Here's how the part is built. I have some questions about the finished solid (model axes, mm). Face numbers are marked on the shaded views. A direction names the side the tool comes from. Round coordinates to 2 decimals unless told otherwise and drop trailing zeros. Write each loop counter-clockwise with the first axis right and the second up, starting at its lowest first coordinate (ties: lowest second). Pieces come first, ordered by that corner, then holes. Notation, with made-up numbers: (77.25, 10) - (87.25, 10) arc R13 cw to (87.25, 20) - close; hole circle Ø2 at (-37, 2). An arc over 180 degrees is marked (long way). Use one line per item in the form item = value. Start each with the question number.
1. I want a section at A-A, the plane x = 0. List the corners of the cut face in (y, z) for me, plus the area to 3 significant figures.
2. Which directions (+Z, -Z, +X, -X, +Y, -Y) give clear straight access to the entire face, cutting with the end or side of a thin tool? Please do the marked faces 1 and 2.
3. I want a section at C-C, the plane z = 3. List the corners of the cut face in (x, y) for me, plus the area to 3 significant figures.
4. Will these pins go through, and if not, where does the flat tip stop? pin 1 (1.5 mm diameter, centred on x = 6.5, y = -6, fed in from +Z); pin 2 (5 mm diameter, centred on y = -7, z = 3, fed in from -X); pin 3 (1.5 mm diameter, centred on x = 1, z = 2.5, fed in from +Y).
5. If I drill on line 1 along X through (y, z) = (0.25, 3.75); line 2 along Z through (x, y) = (-1.75, -12); line 3 along Y through (x, z) = (-1.25, 3.75), over which ranges is the centre line in solid material (lowest first)?
6. I want a section at B-B, the plane y = 0. List the corners of the cut face in (x, z) for me, plus the area to 3 significant figures.
7. We'd pull the mould along Y, two halves only. Please class the marked faces 3, 4 and 5: +Y half, -Y half, draft (parallel to the pull), parting line (faces both ways), or undercut.
8. I want a section at D-D, the plane x = 3. List the corners of the cut face in (y, z) for me, plus the area to 3 significant figures.
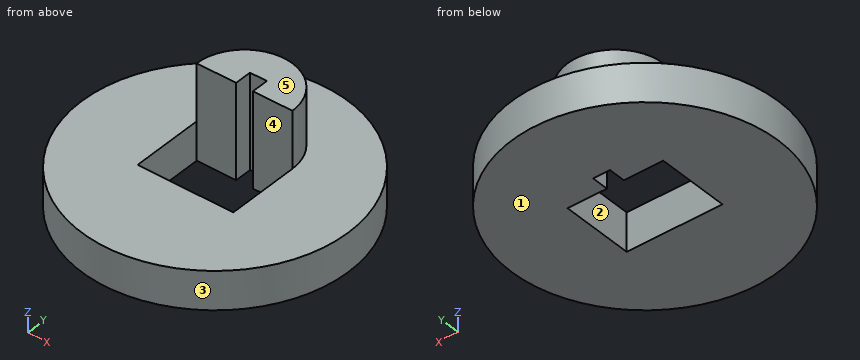
```python
from build123d import *

# Parameters (mm, degrees)
F0_R     = 15
F0_W     = 10.795
F0_H     = 8.128
F1_DEPTH = 4.318
F2_W     = 1.905
F2_H     = 1.905
F3_DEPTH = 25.4
F5_DEPTH = 6.35


with BuildPart() as f1:
    # F0 (on Top) → F1 (new body)
    with BuildSketch(Plane.XY):
        Circle(F0_R)
        Rectangle(F0_W, F0_H, mode=Mode.SUBTRACT)
    extrude(amount=F1_DEPTH)

    # F2 (on face) → F3 (cut)
    with BuildSketch(Plane.XY.offset(4.318)):
        with Locations((0, 5.0165)):
            Rectangle(F2_W, F2_H)
    extrude(amount=-F3_DEPTH, mode=Mode.SUBTRACT)

    # F4 (on face) → F5 (join)
    with BuildSketch(Plane.XY.offset(4.318)):
        with BuildLine():
            Line((0.9525, 4.064), (5.3975, 4.064))
            ThreePointArc((5.3975, 4.064), (0, 9.4615), (-5.3975, 4.064))
            Line((-5.3975, 4.064), (-0.9525, 4.064))
            Line((-0.9525, 4.064), (-0.9525, 5.969))
            Line((-0.9525, 5.969), (0.9525, 5.969))
            Line((0.9525, 5.969), (0.9525, 4.064))
        make_face()
    extrude(amount=F5_DEPTH)


solid = f1.part
```
Model answer:
q1.outline = (-15, 0) - (-4.06, 0) - (-4.06, 4.32) - (-15, 4.32) - close; (5.97, 0) - (15, 0) - (15, 4.32) - (9.46, 4.32) - (9.46, 10.67) - (5.97, 10.67) - close
q1.area = 108 mm2
q2.face_1 = -Z, +X, -X, +Y, -Y
q2.face_2 = +Z, -Z
q3.outline = circle Ø30 at (0, 0); hole (-5.4, -4.06) - (5.4, -4.06) - (5.4, 4.06) - (0.95, 4.06) - (0.95, 5.97) - (-0.95, 5.97) - (-0.95, 4.06) - (-5.4, 4.06) - close
q3.area = 615 mm2
q4.pin_1 = 4.32
q4.pin_2 = -14.31
q4.pin_3 = 15
q5.line_1 = -15 to -5.4, 5.4 to 15
q5.line_2 = 0 to 4.32
q5.line_3 = -14.95 to -4.06, 4.06 to 14.95
q6.outline = (-15, 0) - (-5.4, 0) - (-5.4, 4.32) - (-15, 4.32) - close; (5.4, 0) - (15, 0) - (15, 4.32) - (5.4, 4.32) - close
q6.area = 82.9 mm2
q7.face_3 = parting line
q7.face_4 = undercut
q7.face_5 = draft
q8.outline = (-14.7, 0) - (-4.06, 0) - (-4.06, 4.32) - (-14.7, 4.32) - close; (4.06, 0) - (14.7, 0) - (14.7, 4.32) - (8.55, 4.32) - (8.55, 10.67) - (4.06, 10.67) - close
q8.area = 120 mm2
